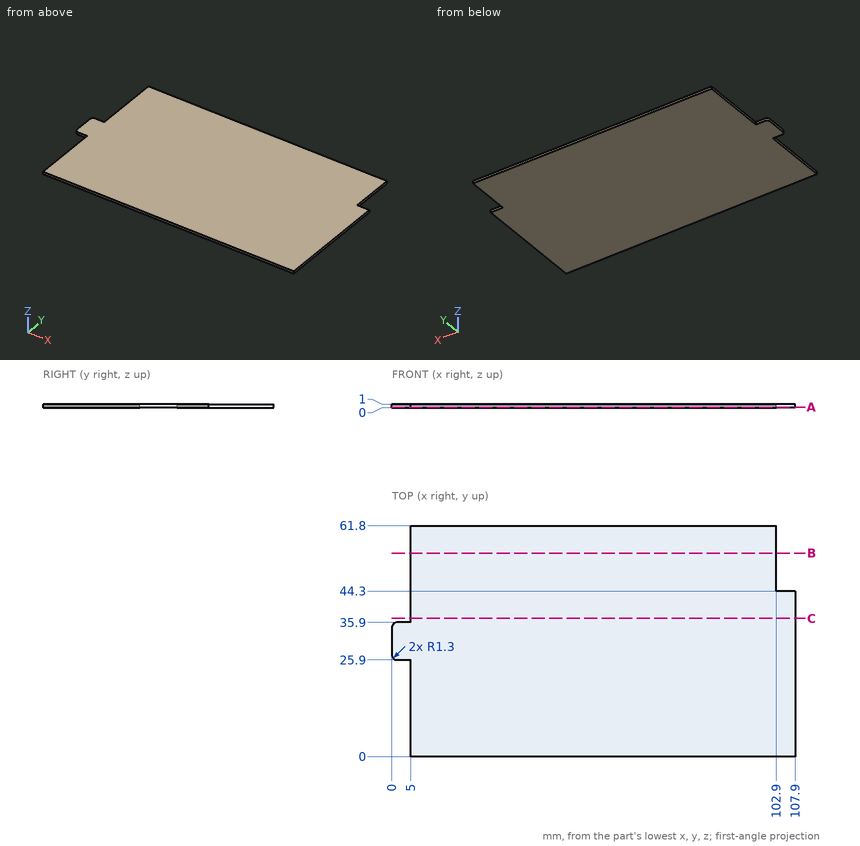
Source: three-view drawing plus pictorial views. Frame: mm from the lowest corner of the part. Give positions to 0.01 mm unless a question says otherwise; leave off trailing zeros. Write each loop counter-clockwise with the first axis right and the second up, starting at its lowest first coordinate (ties: lowest second). Pieces come first, ordered by that corner, then holes.
(1) Cut plane C-C, the plane y = 37. Return loops of the section in (x, z), then the cut area to 3 significant figures.
(2) Cut plane B-B, the plane y = 54.5. Return loops of the section in (x, z).
(3) Ray query, line 1 (X direction, y = 54.5, z = 0.7); line 2 (X direction, y = 36.5, z = 0.85). Return the intervals inside material, ascending.
(4) Cut plane A-A, the plane z = 0.15. Return loops of the section in (x, y).
(5) First-contact query: P1, Ø0.5, axis at y = 52, z = 0.5, coming from the -X side. Flat tip, straight axial feed; report the tip coordinate or a pass-through.
Values follow:
1. outline: (5, 0) - (107.9, 0) - (107.9, 1) - (5, 1) - close
1. area: 103 mm2
2. outline: (5, 0) - (102.9, 0) - (102.9, 1) - (5, 1) - close
3. line 1: x = 5 to 102.9
3. line 2: x = 5 to 107.9
4. outline: (0, 27.2) arc R1.3 ccw to (1.3, 25.9) - (5, 25.9) - (5, 0) - (107.9, 0) - (107.9, 44.3) - (102.9, 44.3) - (102.9, 61.8) - (5, 61.8) - (5, 35.9) - (1.3, 35.9) arc R1.3 ccw to (0, 34.6) - close
5. P1: stops at x = 5
